Read the model definition and answer for the solid it produces. Units are mm, in the model's axes. A direction names the side the tool comes from. Round coordinates to 2 decimals unless told otherwise and drop trailing zeros. Order: outer loops, then holes, each group sorted by start corner. A loop starts at its lowest first (then second) coordinate and runs counter-clockwise, first axis right, second up. Notation, with made-up numbers: (28, 12) -> (84, 12) arc R19 cw to (84, 16) -> close; hole circle Ø10 at (88.5, 21.25). An arc over 180 degrees is marked (long way). Use a Markdown table: item, result. Add a question column.
1. Section C-C, the plane x = 0 is taken. Give the vertices of the cut face in (y, z), then the cut area to 3 significant figures.
2. Section A-A, the plane x = -20 is taken. Give the vertices of the cut face in (y, z), then the cut area to 3 significant figures.
3. Section D-D, the plane y = -20 is taken. Give the vertices of the cut face in (x, z), then the cut area to 3 significant figures.
4. Given pin 1 (8 mm diameter, centred on x = 10, y = 0.5, fed in from +Z); pin 2 (14.5 mm diameter, centred on x = -60, y = 1.03, fed in from +Z); pin 3 (2 mm diameter, centred on x = -74, z = 23, fed in from +Y); pin 4 (4 mm diameter, centred on x = -28.5, z = 7.5, fed in from +Y), each flat-ended and moving along its own axis, determine where each tip first touches the part or whether it passes through.
5. Section B-B, the plane z = 14.5 is taken. Give the vertices of the cut face in (x, y), then the cut area to 3 significant figures.
6. For faces 5 (the face through (-77, 31, 23)), 6 (the face through (57, 0, 23)), 7 (the face through (38.959, 24.967, 1.479)), determine the directions among +Z, -Z, +X, -X, +Y, -Y from which every point of the face is accessible in a straight line to the end or side of a thin tool.
7. The mould has two halves that part along X. Classify faces 1 (the face through (-80, 2, 21)), 2 (the face through (-11, 2, 0)), 3 (the face through (60, 1, 21)), 4 (the face through (28.5, -28.44, 27.05)): +X half, -X half, draft (parallel to the pull), parting line (faces both ways), or undercut.
8. Consider L1, parallel to Y at x = -40, z = 0.9; L2, parallel to X at y = -1.5, z = 23; L3, parallel to Y at x = -17.5, z = 21. Determine where each line is inside the solid, lowest interval first. Write a range as [from, to].
```python
from build123d import *

# Parameters (mm, degrees)
F0_R     = 8
F1_DEPTH = 3
F2_W     = 3
F2_H     = 3
F2_W_2   = 134
F3_DEPTH = 40
F4_W     = 3
F4_H     = 40
F5_DEPTH = 134
F6_W     = 126
F6_H     = 3
F7_DEPTH = 40
F8_R     = 1.5
F9_DEPTH = 3


with BuildPart() as f1:
    # F0 (on Top) → F1 (new body)
    with BuildSketch(Plane.XY):
        Polygon((-60, 33.034884), (-80, 33.034884), (-80, 18.034884), (-80, 0.034884), (-80, -2.965116), (-80, -17.965116), (-80, -29.965116), (60, -29.965116), (60, -24.965116), (60, -14.965116), (60, -9.965116), (60, -4.965116), (60, 0.034884), (60, 18.034884), (60, 33.034884), (40, 33.034884), (20, 33.034884), (0, 33.034884), (-20, 33.034884), (-40, 33.034884), align=None)
        with Locations((-40, -14.965116)):
            Circle(F0_R, mode=Mode.SUBTRACT)
        with Locations((0, -14.965116)):
            Circle(F0_R, mode=Mode.SUBTRACT)
        with Locations((40, -14.965116)):
            Circle(F0_R, mode=Mode.SUBTRACT)
        with Locations((-60, 1.034884)):
            Circle(F0_R, mode=Mode.SUBTRACT)
        with Locations((-20, 1.034884)):
            Circle(F0_R, mode=Mode.SUBTRACT)
        with Locations((-40, 17.034884)):
            Circle(F0_R, mode=Mode.SUBTRACT)
        with Locations((20, 1.034884)):
            Circle(F0_R, mode=Mode.SUBTRACT)
        with Locations((0, 17.034884)):
            Circle(F0_R, mode=Mode.SUBTRACT)
        with Locations((40, 17.034884)):
            Circle(F0_R, mode=Mode.SUBTRACT)
    extrude(amount=F1_DEPTH)

    # F2 (on face) → F3 (join)
    with BuildSketch(Plane.XY.offset(3)):
        with Locations((-78.5, -28.465116)):
            Rectangle(F2_W, F2_H)
        with Locations((-10, -28.465116)):
            Rectangle(F2_W_2, F2_H)
        Polygon((-80, 30.034884), (-80, -26.965116), (-77, -26.965116), (-77, 33.034884), (-80, 33.034884), align=None)
        with Locations((58.5, -28.465116)):
            Rectangle(F2_W, F2_H)
        Polygon((57, 33.034884), (57, -26.965116), (60, -26.965116), (60, 30.034884), (60, 33.034884), align=None)
    extrude(amount=F3_DEPTH)

    # F4 (on face) → F5 (join)
    with BuildSketch(Plane.YZ.offset(-77)):
        with Locations((28.334884, 23)):
            Rectangle(F4_W, F4_H)
    extrude(amount=F5_DEPTH)

    # F6 (on face) → F7 (cut)
    with BuildSketch(Plane.XY.offset(43)):
        with Locations((-10, 28.334884)):
            Rectangle(F6_W, F6_H)
    extrude(amount=-F7_DEPTH, mode=Mode.SUBTRACT)

    # F8 (on face) → F9 (cut)
    with BuildSketch(Plane(origin=(0, -26.965116, 0), x_dir=(-1, 0, 0), z_dir=(0, 1, 0))):
        with Locations((47, 26.988985)):
            Circle(F8_R)
        with Locations((-27, 26.988985)):
            Circle(F8_R)
        with Locations((10, 26.988985)):
            Circle(F8_R)
    extrude(amount=-F9_DEPTH, mode=Mode.SUBTRACT)


solid = f1.part
```
Verdict:
| question | item | result |
|---|---|---|
| 1 | outline | (-29.97, 0) -> (-22.97, 0) -> (-22.97, 3) -> (-26.97, 3) -> (-26.97, 43) -> (-29.97, 43) -> close; (-6.97, 0) -> (9.03, 0) -> (9.03, 3) -> (-6.97, 3) -> close; (25.03, 0) -> (33.03, 0) -> (33.03, 3) -> (25.03, 3) -> close |
| 1 | area | 213 mm2 |
| 2 | outline | (-29.97, 0) -> (-6.97, 0) -> (-6.97, 3) -> (-26.97, 3) -> (-26.97, 43) -> (-29.97, 43) -> close; (9.03, 0) -> (33.03, 0) -> (33.03, 3) -> (9.03, 3) -> close |
| 2 | area | 261 mm2 |
| 3 | outline | (-80, 0) -> (-46.22, 0) -> (-46.22, 3) -> (-77, 3) -> (-77, 43) -> (-80, 43) -> close; (-33.78, 0) -> (-6.22, 0) -> (-6.22, 3) -> (-33.78, 3) -> close; (6.22, 0) -> (33.78, 0) -> (33.78, 3) -> (6.22, 3) -> close; (46.22, 0) -> (60, 0) -> (60, 43) -> (57, 43) -> (57, 3) -> (46.22, 3) -> close |
| 3 | area | 548 mm2 |
| 4 | pin 1 | stops at z = 3 |
| 4 | pin 2 | passes through |
| 4 | pin 3 | stops at y = 29.83 |
| 4 | pin 4 | stops at y = -26.97 |
| 5 | outline | (-80, -29.97) -> (60, -29.97) -> (60, 33.03) -> (57, 33.03) -> (57, 29.83) -> (53, 29.83) -> (53, 26.83) -> (57, 26.83) -> (57, -26.97) -> (-77, -26.97) -> (-77, 26.83) -> (-73, 26.83) -> (-73, 29.83) -> (-77, 29.83) -> (-77, 33.03) -> (-80, 33.03) -> close |
| 5 | area | 804 mm2 |
| 6 | face 5 | +Z, +Y |
| 6 | face 6 | +Z |
| 6 | face 7 | +Z, -Z |
| 7 | face 1 | -X half |
| 7 | face 2 | draft |
| 7 | face 3 | +X half |
| 7 | face 4 | undercut |
| 8 | L1 | y = [-29.97, -22.97], [-6.97, 9.03], [25.03, 33.03] |
| 8 | L2 | x = [-80, -77], [57, 60] |
| 8 | L3 | y = [-29.97, -26.97] |
